```python
from build123d import *

# Parameters (mm, degrees)
F1_DEPTH      = 31.75
F2_R          = 0.127
F3_DEPTH      = 56.2093301913
F3_DEPTH_BACK = 56.2093301913
F4_W          = 90.17
F4_H          = 77.47
F5_DEPTH      = 2.54
F6_W          = 90.17
F6_H          = 77.47
F6_W_2        = 87.63
F6_H_2        = 74.93
F7_DEPTH      = 6.35
F11_W         = 7.62
F11_H         = 3.175
F12_DEPTH     = 79.756
F14_R         = 2.921
F14_R_2       = 2.286
F15_DEPTH     = 6.35
F15_FACE_R    = 2.286
F16_DEPTH     = 12.9286
F17_R         = 2.070357412
F18_DEPTH     = 25.4
F20_R         = 2.286
F21_DEPTH     = 25.4


# Not quite as in the source:
# - a pattern or mirror of a feature is missing from the dataset's text; its kind, count and spacing are read off the source's solid


with BuildPart() as f1:
    # F0 (on Right) → F1 (new body)
    with BuildSketch(Plane.YZ):
        Polygon((-53.9136660383, -18.1264164896), (-39.9723188616, 11.2473889307), (39.9723188616, 11.2473889307), (53.9136660383, -18.1264164896), (56.2083301913, -17.0373267665), (41.5783543673, 13.7873889307), (-41.5783543673, 13.7873889307), (-56.2083301913, -17.0373267665), align=None)
    extrude(amount=F1_DEPTH)

    # F2 (on Front) → F3 (cut, two sides)
    with BuildSketch(Plane.XZ) as f3_sk:
        Polygon((12.8995720297, 13.7873889307), (0, 13.7873889307), (0, -18.1264164896), (19.6673367172, -18.1264164896), (35.7595719397, -19.0736036748), (35.7595719397, -7.4199110855), (17.3968738801, -7.4199110855), align=None)
        with Locations((24.329572916, -1.6249689179)):
            Circle(F2_R)
    extrude(amount=-F3_DEPTH, mode=Mode.SUBTRACT)
    extrude(f3_sk.sketch, amount=F3_DEPTH_BACK, mode=Mode.SUBTRACT)

    # F4 (on face) → F5 (join, through all)
    with BuildSketch(Plane(origin=(0, 0, 11.2473889307), x_dir=(1, 0, 0), z_dir=(0, 0, -1))):
        with Locations((57.9845720297, 0)):
            Rectangle(F4_W, F4_H)
    extrude(amount=-F5_DEPTH)

    # F6 (on face) → F7 (join)
    with BuildSketch(Plane.XY.offset(13.7873889307)):
        with Locations((57.9845720297, 0)):
            Rectangle(F6_W, F6_H)
        with Locations((57.9845720297, 0)):
            Rectangle(F6_W_2, F6_H_2, mode=Mode.SUBTRACT)
    extrude(amount=F7_DEPTH)

    # F11 (on face) → F12 (cut)
    with BuildSketch(Plane(origin=(0, 38.735, 0), x_dir=(-1, 0, 0), z_dir=(0, 1, 0))):
        with Locations((-22.3247860149, 15.3748889307)):
            Rectangle(F11_W, F11_H)
    extrude(amount=-F12_DEPTH, mode=Mode.SUBTRACT)

    # F14 (on face) → F15 (join)
    with BuildSketch(Plane(origin=(0, 39.2749300586, 18.6406026544), x_dir=(-1, 0, 0), z_dir=(0, 0.9034110839, 0.4287754815))):
        with Locations((-24.329572916, -22.4322813106)):
            Circle(F14_R)
        with Locations((-24.329572916, -22.4322813106)):
            Circle(F14_R_2, mode=Mode.SUBTRACT)
    f15 = extrude(amount=-F15_DEPTH)

    # F15_copies: F15 across plane
    add(f15.mirror(Plane(origin=(0, 0, 0), x_dir=(0, 0, -1), z_dir=(0, -1, 0))))

    # F14 (on face) + F15_face (on face) → F16 (cut)
    with BuildSketch(Plane(origin=(0, 39.2749300586, 18.6406026544), x_dir=(-1, 0, 0), z_dir=(0, 0.9034110839, 0.4287754815))):
        with Locations((-24.329572916, -22.4322813106)):
            Circle(F14_R)
        with Locations((-24.329572916, -22.4322813106)):
            Circle(F14_R_2, mode=Mode.SUBTRACT)
    with BuildSketch(Plane(origin=(24.329572916, 46.6004501275, -2.7177921697), x_dir=(1, 0, 0), z_dir=(0, -0.9034110839, -0.4287754815))):
        with Locations((0, 0.004132702)):
            Circle(F15_FACE_R)
        with BuildLine():
            add(Edge.make_bspline(
                [(0.127, 1.2096633209), (0.127, 0.9661745521), (-0.0635, 1.0879189365), (-0.254, 1.2096633209), (-0.0635, 1.3314077053), (0.127, 1.4531520897), (0.127, 1.2096633209)],
                knots=[1.5707963268, 1.5707963268, 1.5707963268, 3.6651914292, 3.6651914292, 5.7595865316, 5.7595865316, 7.853981634, 7.853981634, 7.853981634], degree=2, weights=[1, 0.5, 1, 0.5, 1, 0.5, 1]))
        make_face(mode=Mode.SUBTRACT)
    extrude(amount=F16_DEPTH, dir=(0, 0.9034110839, 0.4287754815), mode=Mode.SUBTRACT)

    # F17 (on face) → F18 (cut)
    with BuildSketch(Plane(origin=(0, 33.5382696761, 15.9178783467), x_dir=(1, 0, 0), z_dir=(0, -0.9034110839, -0.4287754815))):
        with Locations((24.329572916, -22.4322813106)):
            Circle(F17_R)
    extrude(amount=-F18_DEPTH, mode=Mode.SUBTRACT)

    # F20 (on face) → F21 (cut)
    with BuildSketch(Plane(origin=(0, -36.9802659056, 17.5515129313), x_dir=(-1, 0, 0), z_dir=(0, 0.9034110839, -0.4287754815))):
        with Locations((-24.329572916, -22.4322813106)):
            Circle(F20_R)
    extrude(amount=-F21_DEPTH, mode=Mode.SUBTRACT)


solid = f1.part
```
Source: CAD feature listing. Evaluate the final solid. Frame: model axes, mm. A direction names the side the tool comes from. Give positions to 0.01 mm unless a question says otherwise; leave off trailing zeros. Write each loop counter-clockwise with the first axis right and the second up, starting at its lowest first coordinate (ties: lowest second). Pieces come first, ordered by that corner, then holes.
1. Section query D-D (x = 29.5). Return the cut outline in (y, z) (3 decimals).
2. Access query for faces 1 (the face through (57, -1, 11.247)), 2 (the face through (14.17, -1, 17)), 3 (the face through (15.16, 45.22, 3.13)). Directions: +Z, -Z, +X, -X, +Y, -Y. A direction counts if a zero-diameter tool reaches every point of the face in a straight line with its end or side. Return the directions, or none.
3. Section query B-B (z = 4.75). Return the cut outline in (x, y).
4. Pull-direction query (X, two-part tool) for faces 4 (the face through (22.466, 44.34, 2.044)), 5 (the face through (57, -37.465, 17)), 6 (the face through (12.9, -1, 16)); classes: +X half, -X half, draft (parallel to the pull), parting line (faces both ways), or undercut.
5. Section query A-A (x = 58). Return the cut outline in (y, z) (3 decimals).
6. Material intervals for line 1 along X through (y, z) = (-37.5, 14.25); line 2 along X through (y, z) = (-25, 16.5); line 3 along Z through (x, y) = (21, -37.5), sorted ascending.
7. Section query C-C (y = 25). Return the cut outline in (x, z).
8. First-contact query: pin 1 (6 mm diameter, centred on x = 73.5, z = 15.5, fed in from +Y) (3 decimals); pin 2 (0.6 mm diameter, centred on x = 13, z = 13, fed in from +Y); pin 3 (3 mm diameter, centred on x = 72, z = 18.5, fed in from -Y) (3 decimals). Flat tips, straight axial feed; report the tip coordinate or a pass-through.
Output values:
1. outline: (-51.644, -7.42) - (-48.832, -7.42) - (-39.972, 11.247) - (39.972, 11.247) - (48.832, -7.42) - (51.644, -7.42) - (41.578, 13.787) - (38.735, 13.787) - (38.735, 20.137) - (37.465, 20.137) - (37.465, 13.787) - (-37.465, 13.787) - (-37.465, 20.137) - (-38.735, 20.137) - (-38.735, 13.787) - (-41.578, 13.787) - close
2. face 1: -Z, +X, -X
2. face 2: +Z
2. face 3: -Z, -X, +Y
3. outline: (14.82, -45.87) - (31.75, -45.87) - (31.75, -43.06) - (14.82, -43.06) - close; (14.82, 43.06) - (31.75, 43.06) - (31.75, 45.87) - (14.82, 45.87) - close
4. face 4: draft
4. face 5: undercut
4. face 6: -X half
5. outline: (-38.735, 11.247) - (38.735, 11.247) - (38.735, 20.137) - (37.465, 20.137) - (37.465, 13.787) - (-37.465, 13.787) - (-37.465, 20.137) - (-38.735, 20.137) - close
6. line 1: x = 12.9 to 18.51, 26.13 to 103.07
6. line 2: x = 12.9 to 14.17, 101.8 to 103.07
6. line 3: z = 11.25 to 13.79, 16.96 to 20.14
7. outline: (12.9, 11.25) - (103.07, 11.25) - (103.07, 20.14) - (101.8, 20.14) - (101.8, 13.79) - (14.17, 13.79) - (14.17, 20.14) - (12.9, 20.14) - close
8. pin 1: stops at y = 38.735
8. pin 2: stops at y = 42.08
8. pin 3: stops at y = -38.735
